from build123d import *

# Parameters (mm, degrees)
SKETCH_1_R             = 6
EXTRUDE_1_DEPTH        = 20
SKETCH_2_R             = 5
EXTRUDE_2_DEPTH        = 16
EXTRUDE_START          = 25
SKETCH_3_R             = 5
EXTRUDE_3_DEPTH        = 25
HOLE_WIZARD_M5_1_D     = 4.2
HOLE_WIZARD_M5_1_DEPTH = 12.4
HOLE_WIZARD_M5_1_TIP   = 1.2618073
HOLE_WIZARD_M5_2_D     = 4.2
HOLE_WIZARD_M5_2_DEPTH = 12.4
HOLE_WIZARD_M5_2_TIP   = 1.2618073


with BuildPart() as part:
    # 草图1 → 凸台-拉伸1 (new body)
    with BuildSketch(Plane.XY):
        Circle(SKETCH_1_R)
    extrude(amount=EXTRUDE_1_DEPTH)

    # 草图2 → 凸台-拉伸2 (add)
    with BuildSketch(Plane.XY.offset(20)):
        Circle(SKETCH_2_R)
    extrude(amount=EXTRUDE_2_DEPTH)

    # 草图3 → 凸台-拉伸3 (add)
    with BuildSketch(Plane(origin=(0, 0, 0), x_dir=(-1, 0, 0), z_dir=(0, 0, -1)).offset(EXTRUDE_START)):
        with Locations(Location((0, 0, 0), (0, 0, 180))):
            Circle(SKETCH_3_R)
    extrude(amount=-EXTRUDE_3_DEPTH)

    # M5 螺纹孔1
    with Locations(Plane(origin=(0, 0, -25), x_dir=(-1, 0, 0), z_dir=(0, 0, -1))):
        with Locations((0, 0)):
            Hole(HOLE_WIZARD_M5_1_D / 2, depth=HOLE_WIZARD_M5_1_DEPTH)
            with Locations((0, 0, -(HOLE_WIZARD_M5_1_DEPTH + HOLE_WIZARD_M5_1_TIP / 2))):  # 118° drill point
                Cone(0, HOLE_WIZARD_M5_1_D / 2, HOLE_WIZARD_M5_1_TIP, mode=Mode.SUBTRACT)

    # M5 螺纹孔2
    with Locations(Plane.XY.offset(36)):
        with Locations((0, 0)):
            Hole(HOLE_WIZARD_M5_2_D / 2, depth=HOLE_WIZARD_M5_2_DEPTH)
            with Locations((0, 0, -(HOLE_WIZARD_M5_2_DEPTH + HOLE_WIZARD_M5_2_TIP / 2))):  # 118° drill point
                Cone(0, HOLE_WIZARD_M5_2_D / 2, HOLE_WIZARD_M5_2_TIP, mode=Mode.SUBTRACT)


solid = part.part
Geometry check sheet. Reference: the model listing, model coordinates, mm. A direction names the side the tool comes from. Round coordinates to 2 decimals unless told otherwise and drop trailing zeros. Order: outer loops, then holes, each group sorted by start corner. A loop starts at its lowest first (then second) coordinate and runs counter-clockwise, first axis right, second up. Notation, with made-up numbers: M 46,29.5 L 72,29.5 A14 ccw 72,43.5 Z; hole C 75.25,17.25 d3. An arc over 180 degrees is marked long. Answer in a Markdown table with one row per item.
(1) Draft check along X on faces 1 (the face through (-4, 4, 20)), 2 (the face through (-5, 0, -13)), 3 (the face through (-2.003, 0.631, 29.713)). Enter one of: released by +X, released by -X, zero draft, split by the parting line, or undercut.
Responses:
| item | result |
|---|---|
| face 1 | zero draft |
| face 2 | split by the parting line |
| face 3 | undercut |
(2) Scan lines: probe 1 along Y at (x, z) = (0, 30.25); probe 2 along Z at (x, y) = (-5.5, 2.25); probe 3 along Y at (x, z) = (-1.25, 31.5). Record each from-to range of solid material in increasing order. Write a range as from..to.
Responses:
| item | result |
|---|---|
| probe 1 | y = -5..-2.1, 2.1..5 |
| probe 2 | z = 0..20 |
| probe 3 | y = -4.84..-1.69, 1.69..4.84 |
(3) Sectioned sample at D-D, the plane z = -6. Record the cut outline in (x, y), and give its area (3 significant figures).
Responses:
| item | result |
|---|---|
| outline | C 0,0 d10 |
| area | 78.5 mm² |
(4) Sectioned sample at B-B, the plane z = -20.5. Record the cut outline in (x, y).
Responses:
| item | result |
|---|---|
| outline | C 0,0 d10; hole C 0,0 d4.2 |
(5) Sectioned sample at C-C, the plane z = 13. Record the cut outline in (x, y), and give its area (3 significant figures).
Responses:
| item | result |
|---|---|
| outline | C 0,0 d12 |
| area | 113 mm² |
(6) Go/stop test with flat-tipped pins: P1, Ø6, axis at y = -3.5, z = -9.5, coming from the +X side; P2, Ø2.5, axis at x = 0, y = 0, coming from the -Z side; P3, Ø6, axis at y = -4, z = 29, coming from the +X side. Record where each tip stops, or that it passes through.
Responses:
| item | result |
|---|---|
| P1 | stops at x = 4.97 |
| P2 | stops at z = -12.09 |
| P3 | stops at x = 4.9 |
(7) Sectioned sample at A-A, the plane y = -3.25. Record the cut outline in (x, z), and give its area (3 significant figures).
Responses:
| item | result |
|---|---|
| outline | M -5.04,0 L -3.8,0 L -3.8,-25 L 3.8,-25 L 3.8,0 L 5.04,0 L 5.04,20 L 3.8,20 L 3.8,36 L -3.8,36 L -3.8,20 L -5.04,20 Z |
| area | 513 mm² |
(8) Tool access check on faces 4 (the face through (-4, 4, 0)), 5 (the face through (-1.08, -4.88, 27.89)), 6 (the face through (1, -2.2, 36)). Record the directions out of +Z, -Z, +X, -X, +Y, -Y that give a thin tool (end or side, any length) a straight path to the whole face; none if there is none.
Responses:
| item | result |
|---|---|
| face 4 | -Z |
| face 5 | +Z |
| face 6 | +Z, +X, -X, +Y, -Y |
